from build123d import *

# Parameters (mm, degrees)
F1_DEPTH = 10
F2_R     = 5
F3_R     = 4.99999
F5_R     = 4
F6_R     = 2
F7_DEPTH = 10


# Not quite as in the source:
# - two fillets or chamfers of one size are made in one step
# - a fillet or chamfer is up to 0.001 mm smaller than in the source, because OpenCascade refuses the exact size


with BuildPart() as f1:
    # F0 (on Top) → F1 (new body)
    with BuildSketch(Plane.XY):
        Polygon((0, 70.9848281697), (0, 0), (36, 0), (47.5, 0), (47.5, 14.3951736391), (42.5, 14.3951736391), (42.5, 10), (36, 10), (10, 10), (10, 61), (26.8777515739, 61), (31, 61), (31, 56.9848281697), (36, 56.9848281697), (36, 70.9848281697), align=None)
    extrude(amount=F1_DEPTH)

    # F2
    f2_edges = [f1.edges().sort_by_distance(p)[0] for p in [
        (0, 0, 5),
        (0, 70.984828, 5),
    ]]
    fillet(f2_edges, radius=F2_R)

    # F3 (radius 5 in the source; OpenCascade refuses exactly that, so slightly less here)
    f3_edges = [f1.edges().sort_by_distance(p)[0] for p in [
        (10, 10, 5),
        (36, 56.984828, 5),
        (10, 61, 5),
    ]]
    fillet(f3_edges, radius=F3_R)

    # F5
    f5_edges = [f1.edges().sort_by_distance(p)[0] for p in [
        (42.5, 10, 5),
    ]]
    fillet(f5_edges, radius=F5_R)

    # F6 (on face) → F7 (cut, through all)
    with BuildSketch(Plane.XY.offset(10)):
        with Locations((6.6156452522, 64.5774751902)):
            Circle(F6_R)
    extrude(amount=-F7_DEPTH, mode=Mode.SUBTRACT)


solid = f1.part
Geometry: final body of the model. Coordinates: model frame, mm. A direction names the side the tool comes from. Round coordinates to 2 decimals unless told otherwise and drop trailing zeros. Order: outer loops, then holes, each group sorted by start corner. A loop starts at its lowest first (then second) coordinate and runs counter-clockwise, first axis right, second up. Notation, with made-up numbers: (70.25, 2) - (80.25, 2) arc R18 cw to (80.25, 13) - close; hole circle Ø10 at (-35.5, 2.5). An arc over 180 degrees is marked (long way). Write each question's results on one line, items separated by ' | '.
Item 1: Reachability of faces 5 (the cylindrical face through (12, 60, 5)), 6 (the cylindrical face through (41.297, 11.141, 5.07)), 7 (the flat face through (10, 35, 5)), 8 (the flat face through (45, 14.395, 5)) from +Z, -Z, +X, -X, +Y, -Y: full face, straight path, thin tool, end or side. Return the list, or none.
Completed:
face 5: +Z, -Z | face 6: +Z, -Z, +Y | face 7: +Z, -Z, +X | face 8: +Z, -Z, +X, +Y
Item 2: First-contact query: pin 1 Ø5 at (y, z) = (27.5, 2.5) entering from +X; pin 2 Ø8 at (x, y) = (13, 58.5) entering from -Z; pin 3 Ø2.5 at (x, z) = (45.5, 2.5) entering from +Y. Flat tips, straight axial feed; report the tip coordinate or a pass-through.
Completed:
pin 1: x = 10 | pin 2: z = 0 | pin 3: y = 14.4
Item 3: Material intervals for line 1 along Y through (x, z) = (24, 8.25); line 2 along X through (y, z) = (39.5, 9.25); line 3 along Y through (x, z) = (11, 3), sorted ascending. Write a range as [from, to].
Completed:
line 1: [0, 10], [61, 70.98] | line 2: [0, 10] | line 3: [0, 12], [59, 70.98]
Item 4: Section A-A, the plane x = 24.5. Return the cut outline in (y, z), and give its area (3 significant figures).
Completed:
outline: (0, 0) - (10, 0) - (10, 10) - (0, 10) - close; (61, 0) - (70.98, 0) - (70.98, 10) - (61, 10) - close | area: 200 mm^2
Item 5: Section C-C, the plane y = 29.5. Return the cut outline in (x, z).
Completed:
outline: (0, 0) - (10, 0) - (10, 10) - (0, 10) - close
Item 6: Section D-D, the plane x = 32. Return the cut outline in (y, z).
Completed:
outline: (0, 0) - (10, 0) - (10, 10) - (0, 10) - close; (57.09, 0) - (70.98, 0) - (70.98, 10) - (57.09, 10) - close
Item 7: Mould query, pull axis X, two halves, no side actions, for faces 1 (the flat face through (23, 61, 5)), 2 (the flat face through (26, 0, 5)), 3 (the flat face through (36, 66, 5)), 4 (the flat face through (31, 59, 5)). Classes: pulls with the +X half, pulls with the -X half, needs draft (parallel to the pull), parting line crosses it, or undercut.
Completed:
face 1: undercut | face 2: needs draft | face 3: pulls with the +X half | face 4: undercut
